Part model, mm, in its own coordinate system. A direction names the side the tool comes from. Coordinates: 2 decimals unless noted, no trailing zeros. Order: outer loops, then holes, each group sorted by start corner. A loop starts at its lowest first (then second) coordinate and runs counter-clockwise, first axis right, second up.
1) Pin check, flat tips, straight feed: pin 1 Ø2 at (x, y) = (1, 6) entering from -Z; pin 2 Ø2 at (x, z) = (2, 1) entering from +Y; pin 3 Ø1.5 at (y, z) = (4, 0.5) entering from -X. Stop position of each tip, or through.
2) Cut at D-D (x = 1.7). List the corners of the cut face in (y, z) (3 decimals), and give its area (3 significant figures).
3) Wall check: L1, parallel to X at y = 3.25, z = -0.05; L2, parallel to Y at x = -0.5, z = -2.2; L3, parallel to Y at x = -0.35, z = 0.45. Give the ranges that are in metal, low to high.
4) Mould opens along Z. For faces 1 (the flat face through (0, 8.9, 0)), 2 (the cylindrical face through (-1.45, 5.73, -0.06)), 3 (the flat face through (0, 1, -1.27)) say: +Z half, -Z half, draft (parallel to the pull), parting line (faces both ways), or undercut.
5) Cut at B-B (y = 7). List the corners of the cut face in (x, z), and give its area (3 significant figures).
6) Cut at A-A (x = 0). List the corners of the cut face in (y, z) (3 decimals).
7) Tool access for faces 4 (the flat face through (0, 2.9, 2)), 5 (the flat face through (0, 1, 1.27)), 6 (the flat face through (1.1, 0, 1.1)): list every direction of +Z, -Z, +X, -X, +Y, -Y with a clear straight run to the whole face (end or side of a thin tool).
8) Cut at C-C (z = -2.1). List the corners of the cut face in (x, y), and give its area (3 significant figures).
```python
from build123d import *

# Parameters (mm, degrees)
SKETCH1_R           = 2.465
BOSS_EXTRUDE1_DEPTH = 2.9
SKETCH2_R           = 1.45
BOSS_EXTRUDE2_DEPTH = 6
CUT_EXTRUDE1_DEPTH  = 1.9
CHAMFER1_SIZE       = 0.25


with BuildPart() as part:
    # Sketch1 → Boss-Extrude1 (new body)
    with BuildSketch(Plane(origin=(0, 0, 0), x_dir=(1, 0, 0), z_dir=(0, 1, 0))):
        Circle(SKETCH1_R)
    extrude(amount=BOSS_EXTRUDE1_DEPTH)

    # Sketch2 → Boss-Extrude2 (add)
    with BuildSketch(Plane(origin=(0, 2.9, 0), x_dir=(1, 0, 0), z_dir=(0, 1, 0))):
        Circle(SKETCH2_R)
    extrude(amount=BOSS_EXTRUDE2_DEPTH)

    # Sketch3 → Cut-Extrude1 (cut)
    with BuildSketch(Plane.XZ):
        Polygon((0.733234842, -1.27), (1.466469684, 0), (0.733234842, 1.27), (-0.733234842, 1.27), (-1.466469684, 0), (-0.733234842, -1.27), align=None)
    extrude(amount=-CUT_EXTRUDE1_DEPTH, mode=Mode.SUBTRACT)

    # Chamfer1
    chamfer1_edges = [part.edges().sort_by_distance(p)[0] for p in [
        (-1.45, 8.9, 0),
    ]]
    chamfer(chamfer1_edges, length=CHAMFER1_SIZE)


solid = part.part
```
Geometry check:
1. pin 1: stops at z = -1.45
1. pin 2: stops at y = 8.86
1. pin 3: stops at x = -1.45
2. outline: (0, -1.785) - (2.9, -1.785) - (2.9, 1.785) - (0, 1.785) - close
2. area: 10.4 mm2
3. L1: x = -1.45 to 1.45
3. L2: y = 0 to 2.9
3. L3: y = 1.9 to 8.9
4. face 1: draft
4. face 2: parting line
4. face 3: undercut
5. outline: circle Ø2.9 at (0, 0)
5. area: 6.61 mm2
6. outline: (0, -2.465) - (2.9, -2.465) - (2.9, -1.45) - (8.65, -1.45) - (8.9, -1.2) - (8.9, 1.2) - (8.65, 1.45) - (2.9, 1.45) - (2.9, 2.465) - (0, 2.465) - (0, 1.27) - (1.9, 1.27) - (1.9, -1.27) - (0, -1.27) - close
7. face 4: +Y
7. face 5: -Y
7. face 6: +Z, -Z, +X, -X, -Y
8. outline: (-1.29, 0) - (1.29, 0) - (1.29, 2.9) - (-1.29, 2.9) - close
8. area: 7.49 mm2
